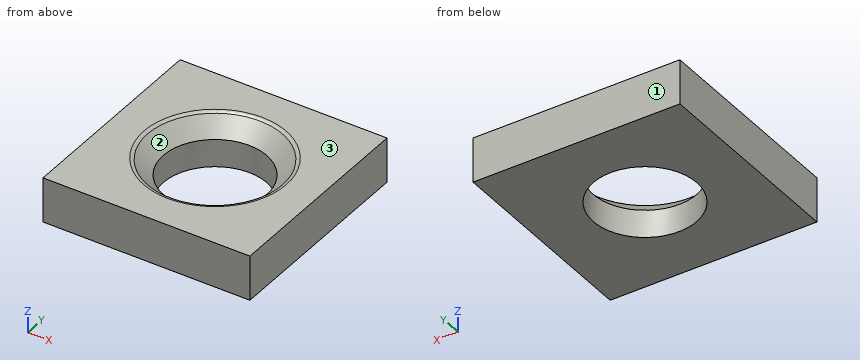
from build123d import *

# Parameters (mm, degrees)
SKETCH1_W           = 60
SKETCH1_H           = 60
SKETCH1_R           = 15
BOSS_EXTRUDE1_DEPTH = 13
CHAMFER1_SIZE       = 5
FILLET1_R           = 1.5


with BuildPart() as part:
    # Sketch1 → Boss-Extrude1 (new body)
    with BuildSketch(Plane.XY):
        Rectangle(SKETCH1_W, SKETCH1_H)
        with Locations(Location((0, 0, 0), (0, 0, 180))):
            Circle(SKETCH1_R, mode=Mode.SUBTRACT)
    extrude(amount=BOSS_EXTRUDE1_DEPTH)

    # Chamfer1
    chamfer1_edges = [part.edges().sort_by_distance(p)[0] for p in [
        (15, 0, 13),
    ]]
    chamfer(chamfer1_edges, length=CHAMFER1_SIZE)

    # Fillet1
    fillet1_edges = [part.edges().sort_by_distance(p)[0] for p in [
        (20, 0, 13),
    ]]
    fillet(fillet1_edges, radius=FILLET1_R)


solid = part.part
Work out the finished part from the listing and answer in its coordinate system (mm). Face numbers are marked on the shaded views. Give positions to 0.01 mm unless a question says otherwise; leave off trailing zeros. Order: outer loops, then holes, each group sorted by start corner. A loop starts at its lowest first (then second) coordinate and runs counter-clockwise, first axis right, second up. Notation, with made-up numbers: (70, 76) -> (114, 76) arc R23 cw to (114, 105) -> close; hole circle Ø2 at (-24.5, 12.5). An arc over 180 degrees is marked (long way). One line per item, written item: value.
Item 1: A flat-ended cylindrical pin translates along its axis: P1, Ø12, axis at x = -10.5, y = -17, coming from the -Z side. Find the tip coordinate at first contact, or state that the pin passes through.
Answer sheet:
P1: z = 0
Item 2: Straight lines are drawn through the part: probe 1 along Y at (x, z) = (0, 5.5); probe 2 along X at (y, z) = (10, 1.75); probe 3 along X at (y, z) = (-1, 5.5). For each, find the intervals that lie inside material, in ascending order.
Answer sheet:
probe 1: -30 to -15, 15 to 30
probe 2: -30 to -11.18, 11.18 to 30
probe 3: -30 to -14.97, 14.97 to 30
Item 3: Determine the mould class of the marked faces 1, 2 and 3 for opening direction Y: released by +Y, released by -Y, zero draft, split by the parting line, or undercut.
Answer sheet:
face 1: released by +Y
face 2: undercut
face 3: zero draft
Item 4: Find section A-A, the plane z = 11.75. Give the vertices of the cut face in (x, y).
Answer sheet:
outline: (-30, -30) -> (30, -30) -> (30, 30) -> (-30, 30) -> close; hole circle Ø37.5 at (0, 0)
Item 5: Find section B-B, the plane y = 0. Give the vertices of the cut face in (x, z), plus the area to 3 significant figures.
Answer sheet:
outline: (-30, 0) -> (-15, 0) -> (-15, 8) -> (-19.56, 12.56) arc R1.5 ccw to (-20.62, 13) -> (-30, 13) -> close; (15, 0) -> (30, 0) -> (30, 13) -> (20.62, 13) arc R1.5 ccw to (19.56, 12.56) -> (15, 8) -> close
area: 365 mm²
Item 6: Find section D-D, the plane z = 3.5. Give the vertices of the cut face in (x, y), plus the area to 3 significant figures.
Answer sheet:
outline: (-30, -30) -> (30, -30) -> (30, 30) -> (-30, 30) -> close; hole circle Ø30 at (0, 0)
area: 2,890 mm²
